Check sheet for the modelled part. Datum: model origin and axes. Units: mm. Face numbers are marked on the shaded views. A direction names the side the tool comes from. Round coordinates to 2 decimals unless told otherwise and drop trailing zeros. Loops run counter-clockwise (first coordinate to the right, second up) from the corner with the lowest first, then second, coordinate; pieces in that order, holes last. Notation, with made-up numbers: (68.25, -37) - (103.25, -37) arc R27 ccw to (103.25, 1) - close; hole circle Ø6 at (59.5, 4). An arc over 180 degrees is marked (long way). Put each result on its own line as item: value.
```python
from build123d import *

# Parameters (mm, degrees)
SKETCH001_R           = 1.9
POCKET_DEPTH          = 4.5
POLARPATTERN_COUNT    = 3
POCKET001_DEPTH       = 1
POCKET002_DEPTH       = 2.2
POLARPATTERN001_COUNT = 3
SKETCH004_R           = 2
POCKET003_DEPTH       = 4


with BuildPart() as part:
    # Sketch → Revolution (revolve)
    with BuildSketch(Plane.XZ):
        Polygon((0, 0), (15, 0), (15, 5), (0, 8), align=None)
    revolve(axis=Axis((0, 0, 0), (0, 0, 1)))

    # Sketch001 → Pocket (cut)
    with BuildSketch(Plane(origin=(0, 0, 0), x_dir=(1, 0, 0), z_dir=(0, 0, -1))):
        with Locations((0, 10)):
            Circle(SKETCH001_R)
    pocket = extrude(amount=-POCKET_DEPTH, mode=Mode.SUBTRACT)

    # PolarPattern: Pocket ×3 about axis
    polarpattern_axis = Axis((0, 0, 0), (0, 0, -1))
    for i in range(1, POLARPATTERN_COUNT):
        add(pocket.rotate(polarpattern_axis, i * 360 / POLARPATTERN_COUNT), mode=Mode.SUBTRACT)

    # Sketch002 → Pocket001 (cut)
    with BuildSketch(Plane(origin=(0, 0, 0), x_dir=(1, 0, 0), z_dir=(0, 0, -1))):
        with BuildLine():
            Line((4.884242, 5.24479), (6.984242, 1.607483))
            Line((6.984242, 1.607483), (13.912445, 5.607483))
            ThreePointArc((13.912445, 5.607483), (12.990381, 7.5), (11.812445, 9.24479))
            Line((4.884242, 5.24479), (11.812445, 9.24479))
        make_face()
    pocket001 = extrude(amount=-POCKET001_DEPTH, mode=Mode.SUBTRACT)

    # Sketch003 → Pocket002 (cut)
    with BuildSketch(Plane(origin=(0, 0, 1), x_dir=(1, 0, 0), z_dir=(0, 0, -1))):
        Polygon((4.884242, 5.24479), (6.984242, 1.607483), (10.448344, 3.607483), (8.34834, 7.244788), align=None)
    pocket002 = extrude(amount=-POCKET002_DEPTH, mode=Mode.SUBTRACT)

    # PolarPattern001: Pocket002, Pocket001 ×3 about axis
    polarpattern001_axis = Axis((0, 0, 1), (0, 0, -1))
    for i in range(1, POLARPATTERN001_COUNT):
        add(pocket002.rotate(polarpattern001_axis, i * 360 / POLARPATTERN001_COUNT), mode=Mode.SUBTRACT)
        add(pocket001.rotate(polarpattern001_axis, i * 360 / POLARPATTERN001_COUNT), mode=Mode.SUBTRACT)

    # Sketch004 → Pocket003 (cut)
    with BuildSketch(Plane(origin=(0, 0, 0), x_dir=(1, 0, 0), z_dir=(0, 0, -1))):
        Circle(SKETCH004_R)
    extrude(amount=-POCKET003_DEPTH, mode=Mode.SUBTRACT)


solid = part.part
```
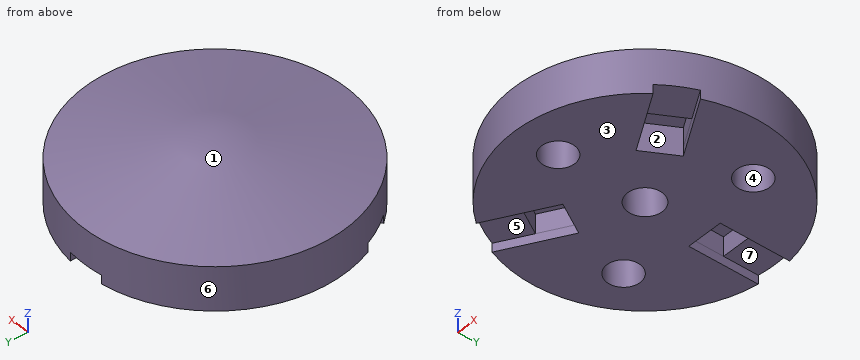
Item 1: Release check for a two-part mould opening along Y. For the marked faces 1, 2, 3 and 4 record: +Y half, -Y half, draft (parallel to the pull), parting line (faces both ways), or undercut.
Filled sheet:
face 1: parting line
face 2: undercut
face 3: draft
face 4: undercut
Item 2: Section check B-B on z = 6. Enter the section's corners in (x, y), then the cut area to 3 significant figures.
Filled sheet:
outline: circle Ø20 at (0, 0)
area: 314 mm²
Item 3: Tool access check on the marked faces 5, 6 and 7. Record the directions out of +Z, -Z, +X, -X, +Y, -Y that give a thin tool (end or side, any length) a straight path to the whole face; none if there is none.
Filled sheet:
face 5: -Z
face 6: +Z, -Z
face 7: -Z, +Y
Item 4: Go/stop test with flat-tipped pins: pin 1 (1.9 mm diameter, centred on x = 9, y = 5.5, fed in from -Z); pin 2 (1.2 mm diameter, centred on x = 0.5, y = 9, fed in from -Z); pin 3 (1.8 mm diameter, centred on y = 9, z = 1.5, fed in from -X) (3 decimals). Record where each tip stops, or that it passes through.
Filled sheet:
pin 1: z = 4.5
pin 2: z = 3.2
pin 3: x = -12.625
Item 5: Thickness scan on line 1 (Y direction, x = 0, z = 2.05); line 2 (Y direction, x = -1.5, z = 1.75); line 3 (Y direction, x = 7.25, z = 1.25). Record the ranges inside material, lowest first. Write a range as from..to.
Filled sheet:
line 1: -15..-11.9, -8.1..-2, 2..6.85, 10.85..15
line 2: -14.92..-11.17, -8.83..-1.32, 1.32..6.85, 10.85..14.92
line 3: -13.13..-6.61, -1.76..3.73, 6.27..13.13
Item 6: Section check A-A on z = 2.25. Enter the section's corners in (x, y).
Filled sheet:
outline: circle Ø30 at (0, 0); hole circle Ø3.8 at (-8.66, 5); hole (-10.45, -3.61) - (-8.35, -7.24) - (-4.88, -5.24) - (-6.98, -1.61) - close; hole (-2.1, 6.85) - (2.1, 6.85) - (2.1, 10.85) - (-2.1, 10.85) - close; hole circle Ø4 at (0, 0); hole circle Ø3.8 at (0, -10); hole (4.88, -5.24) - (8.35, -7.24) - (10.45, -3.61) - (6.98, -1.61) - close; hole circle Ø3.8 at (8.66, 5)
